For this review, take the finished solid that the model builds, in its own axes (mm). Face numbers are marked on the shaded views. A direction names the side the tool comes from. Round coordinates to 2 decimals unless told otherwise and drop trailing zeros. Write each loop counter-clockwise with the first axis right and the second up, starting at its lowest first coordinate (ties: lowest second). Pieces come first, ordered by that corner, then holes. Notation, with made-up numbers: (-29.75, 27) - (-15.75, 27) arc R17 cw to (-15.75, 58) - close; hole circle Ø3 at (36.25, 47.25). An arc over 180 degrees is marked (long way). One line per item, written item: value. Start each with the question number.
Q1. Mouldability with a two-part tool opening along X and no side actions: class the marked faces 1, 2 and 3 as +X half, -X half, draft (parallel to the pull), parting line (faces both ways), or undercut.
Q2. Add section C-C on y = 32.5. Write out the cut boundary in (x, z).
Q3. Add section A-A on z = 0. Write out the cut boundary in (x, y), and give its area (3 significant figures).
Q4. For probe 1 along Z at (x, y) = (0, 19); probe 2 along X at (y, z) = (34, 0), list the stretches that pass through material, from the lowest coordinate up.
Q5. Add section D-D on y = 7.5. Write out the cut boundary in (x, z).
Q6. Add section B-B on x = 0. Write out the cut boundary in (y, z).
Q7. Clearance check with flat-ended pins moving along their axes: pin 1 Ø1 at (x, z) = (-40, -33.5) entering from +Y; pin 2 Ø19 at (x, z) = (-4.5, 2.5) entering from +Y; pin 3 Ø5 at (x, y) = (-24, 36.5) entering from +Z; pin 4 Ø4 at (x, z) = (12, 40) entering from +Y. State where each tip first meets the part, or that it passes through.
Q8. Tool access review of the marked faces 4 and 5: name each direction out of +Z, -Z, +X, -X, +Y, -Y from which nothing blocks a thin tool from reaching the whole face with its end or side.
```python
from build123d import *

# Parameters (mm, degrees)
SKETCH1_W           = 50.8
SKETCH1_H           = 25.4
SKETCH2_R           = 6.35
CUT_EXTRUDE1_DEPTH  = 26.4
SKETCH4_R           = 50.8
SKETCH4_R_2         = 44.45
BOSS_EXTRUDE1_DEPTH = 12.7
SKETCH6_R           = 19.05
BOSS_EXTRUDE2_DEPTH = 38.1
SKETCH7_R           = 12.7
BOSS_EXTRUDE3_DEPTH = 19.05
SKETCH8_R           = 7.112
CUT_EXTRUDE2_DEPTH  = 83.55


with BuildPart() as part:
    # Sketch1 → Revolve1 (revolve)
    with BuildSketch(Plane.XY):
        with Locations((25.4, 12.7)):
            Rectangle(SKETCH1_W, SKETCH1_H)
    revolve(axis=Axis((0, 25.4, 0), (0, -1, 0)))

    # Sketch2 → Cut-Extrude1 (cut, through all)
    with BuildSketch(Plane(origin=(0, 25.4, 0), x_dir=(1, 0, 0), z_dir=(0, 1, 0))):
        with Locations((29.337, 0)):
            Circle(SKETCH2_R)
        with Locations((0, -29.337)):
            Circle(SKETCH2_R)
        with Locations((-29.337, 0)):
            Circle(SKETCH2_R)
        with Locations((0, 29.337)):
            Circle(SKETCH2_R)
    extrude(amount=-CUT_EXTRUDE1_DEPTH, mode=Mode.SUBTRACT)

    # Sketch4 → Boss-Extrude1 (add)
    with BuildSketch(Plane(origin=(0, 25.4, 0), x_dir=(1, 0, 0), z_dir=(0, 1, 0))):
        Circle(SKETCH4_R)
        Circle(SKETCH4_R_2, mode=Mode.SUBTRACT)
    extrude(amount=BOSS_EXTRUDE1_DEPTH)

    # Sketch6 → Boss-Extrude2 (add)
    with BuildSketch(Plane(origin=(0, 25.4, 0), x_dir=(1, 0, 0), z_dir=(0, 1, 0))):
        Circle(SKETCH6_R)
    extrude(amount=BOSS_EXTRUDE2_DEPTH)

    # Sketch7 → Boss-Extrude3 (add)
    with BuildSketch(Plane(origin=(0, 63.5, 0), x_dir=(1, 0, 0), z_dir=(0, 1, 0))):
        Circle(SKETCH7_R)
    extrude(amount=BOSS_EXTRUDE3_DEPTH)

    # Sketch8 → Cut-Extrude2 (cut, through all)
    with BuildSketch(Plane(origin=(0, 82.55, 0), x_dir=(1, 0, 0), z_dir=(0, 1, 0))):
        Circle(SKETCH8_R)
    extrude(amount=-CUT_EXTRUDE2_DEPTH, mode=Mode.SUBTRACT)


solid = part.part
```
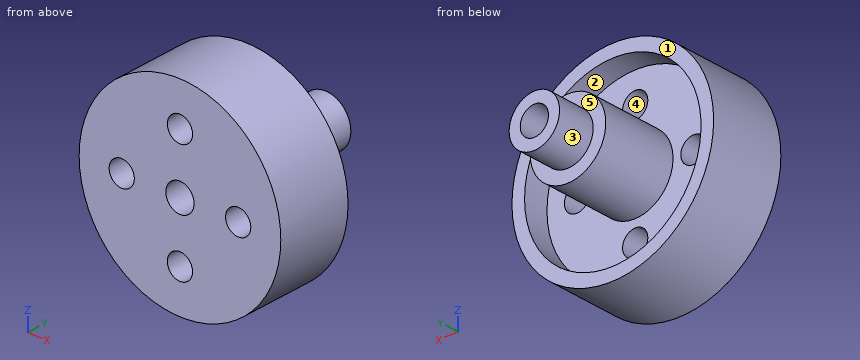
Result set:
1. face 1: draft
1. face 2: undercut
1. face 3: parting line
2. outline: circle Ø101.6 at (0, 0); circle Ø38.1 at (0, 0); hole circle Ø88.9 at (0, 0); hole circle Ø14.22 at (0, 0)
3. outline: (-50.8, 0) - (-35.69, 0) - (-35.69, 25.4) - (-44.45, 25.4) - (-44.45, 38.1) - (-50.8, 38.1) - close; (-22.99, 0) - (-7.11, 0) - (-7.11, 82.55) - (-12.7, 82.55) - (-12.7, 63.5) - (-19.05, 63.5) - (-19.05, 25.4) - (-22.99, 25.4) - close; (7.11, 0) - (22.99, 0) - (22.99, 25.4) - (19.05, 25.4) - (19.05, 63.5) - (12.7, 63.5) - (12.7, 82.55) - (7.11, 82.55) - close; (35.69, 0) - (50.8, 0) - (50.8, 38.1) - (44.45, 38.1) - (44.45, 25.4) - (35.69, 25.4) - close
3. area: 2,860 mm^2
4. probe 1: z = -50.8 to -35.69, -22.99 to -7.11, 7.11 to 22.99, 35.69 to 50.8
4. probe 2: x = -50.8 to -44.45, -19.05 to -7.11, 7.11 to 19.05, 44.45 to 50.8
5. outline: circle Ø101.6 at (0, 0); hole circle Ø12.7 at (-29.34, 0); hole circle Ø14.22 at (0, 0); hole circle Ø12.7 at (0, -29.34); hole circle Ø12.7 at (0, 29.34); hole circle Ø12.7 at (29.34, 0)
6. outline: (0, -50.8) - (38.1, -50.8) - (38.1, -44.45) - (25.4, -44.45) - (25.4, -35.69) - (0, -35.69) - close; (0, -22.99) - (25.4, -22.99) - (25.4, -19.05) - (63.5, -19.05) - (63.5, -12.7) - (82.55, -12.7) - (82.55, -7.11) - (0, -7.11) - close; (0, 7.11) - (82.55, 7.11) - (82.55, 12.7) - (63.5, 12.7) - (63.5, 19.05) - (25.4, 19.05) - (25.4, 22.99) - (0, 22.99) - close; (0, 35.69) - (25.4, 35.69) - (25.4, 44.45) - (38.1, 44.45) - (38.1, 50.8) - (0, 50.8) - close
7. pin 1: passes through
7. pin 2: stops at y = 82.55
7. pin 3: stops at z = 46.03
7. pin 4: stops at y = 25.4
8. face 4: +Y, -Y
8. face 5: +Y
